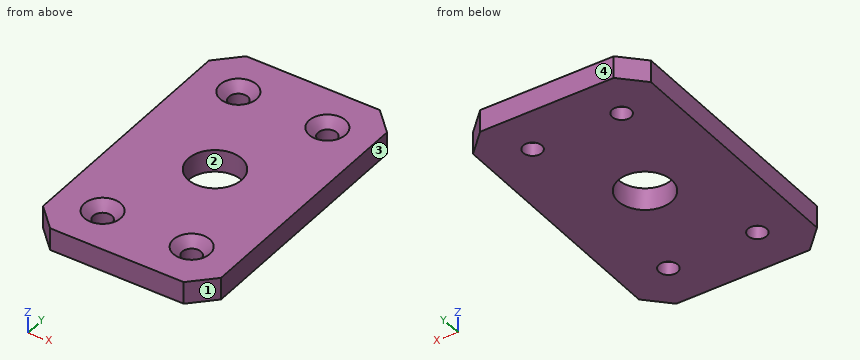
from build123d import *

# Parameters (mm, degrees)
SKETCH_1_W               = 40
SKETCH_1_H               = 65
SKETCH_1_R               = 6
EXTRUDE_1_DEPTH          = 2.5
CUT_EXTRUDE_1_DEPTH      = 39.487010796
CUT_EXTRUDE_1_DEPTH_BACK = 39.487010796
SKETCH_2_R               = 2.1
CHAMFER_1_SIZE           = 2
CHAMFER_2_SIZE           = 5


with BuildPart() as part:
    # 草图1 → 凸台-拉伸1 (new, symmetric)
    with BuildSketch(Plane.XY):
        Rectangle(SKETCH_1_W, SKETCH_1_H)
        Circle(SKETCH_1_R, mode=Mode.SUBTRACT)
    extrude(amount=EXTRUDE_1_DEPTH, both=True)

    # 草图2 → 切除-拉伸1 (cut, two sides: drawn at the far end of the back side and taken through both)
    with BuildSketch(Plane(origin=(0, 0, -2.5), x_dir=(-1, 0, 0), z_dir=(0, 0, -1)).offset(-CUT_EXTRUDE_1_DEPTH_BACK)):
        with Locations((-10, 22.5)):
            Circle(SKETCH_2_R)
        with Locations((10, 22.5)):
            Circle(SKETCH_2_R)
        with Locations((10, -22.5)):
            Circle(SKETCH_2_R)
        with Locations((-10, -22.5)):
            Circle(SKETCH_2_R)
    extrude(amount=CUT_EXTRUDE_1_DEPTH + CUT_EXTRUDE_1_DEPTH_BACK, mode=Mode.SUBTRACT)

    # 倒角1
    chamfer_1_edges = [part.edges().sort_by_distance(p)[0] for p in [
        (12.1, -22.5, 2.5),
        (-7.9, -22.5, 2.5),
        (-7.9, 22.5, 2.5),
        (12.1, 22.5, 2.5),
    ]]
    chamfer(chamfer_1_edges, length=CHAMFER_1_SIZE)

    # 倒角2
    chamfer_2_edges = [part.edges().sort_by_distance(p)[0] for p in [
        (-20, 32.5, 0),
        (20, 32.5, 0),
        (20, -32.5, 0),
        (-20, -32.5, 0),
    ]]
    chamfer(chamfer_2_edges, length=CHAMFER_2_SIZE)


solid = part.part
Check sheet for the modelled part. Datum: model origin and axes. Units: mm. Face numbers are marked on the shaded views. Give positions to 0.01 mm unless a question says otherwise; leave off trailing zeros. Loops run counter-clockwise (first coordinate to the right, second up) from the corner with the lowest first, then second, coordinate; pieces in that order, holes last. Notation, with made-up numbers: M 83,3.25 L 134,3.25 A30 cw 134,35.25 Z; hole C -27,48 d3. An arc over 180 degrees is marked long. Use a Markdown table: item, result. Add a question column.
Q1. Sectioned sample at D-D, the plane z = -1.4. Record the cut outline in (x, y), then the cut area to 3 significant figures.
Q2. Mould release check, pull along Y, two halves, no side actions. Record for the marked faces 1, 2, 3 and 4: pulls with the +Y half, pulls with the -Y half, needs draft (parallel to the pull), parting line crosses it, or undercut.
Q3. Go/stop test with flat-tipped pins: pin 1 (2.5 mm diameter, centred on x = -10, y = -22.5, fed in from -Z); pin 2 (5.5 mm diameter, centred on x = 10, y = 22.5, fed in from -Z). Record where each tip stops, or that it passes through.
Q4. Sectioned sample at B-B, the plane x = -10. Record the cut outline in (y, z).
Q5. Sectioned sample at C-C, the plane y = 0. Record the cut outline in (x, z).
Q6. Scan lines: line 1 along Y through (x, z) = (10, -1.4); line 2 along X through (y, z) = (22.5, -1.75); line 3 along X through (y, z) = (20.5, 1.05). Record each from-to range of solid material in increasing order. Write a range as [from, to].
Q7. Sectioned sample at A-A, the plane x = 0. Record the cut outline in (y, z), then the cut area to 3 significant figures.
Verdict:
| question | item | result |
|---|---|---|
| 1 | outline | M -20,-27.5 L -15,-32.5 L 15,-32.5 L 20,-27.5 L 20,27.5 L 15,32.5 L -15,32.5 L -20,27.5 Z; hole C -10,-22.5 d4.2; hole C -10,22.5 d4.2; hole C 0,0 d12; hole C 10,-22.5 d4.2; hole C 10,22.5 d4.2 |
| 1 | area | 2,380 mm^2 |
| 2 | face 1 | pulls with the -Y half |
| 2 | face 2 | undercut |
| 2 | face 3 | needs draft |
| 2 | face 4 | pulls with the +Y half |
| 3 | pin 1 | through |
| 3 | pin 2 | z = -2.5 |
| 4 | outline | M -32.5,-2.5 L -24.6,-2.5 L -24.6,0.5 L -26.6,2.5 L -32.5,2.5 Z; M -20.4,-2.5 L 20.4,-2.5 L 20.4,0.5 L 18.4,2.5 L -18.4,2.5 L -20.4,0.5 Z; M 24.6,-2.5 L 32.5,-2.5 L 32.5,2.5 L 26.6,2.5 L 24.6,0.5 Z |
| 5 | outline | M -20,-2.5 L -6,-2.5 L -6,2.5 L -20,2.5 Z; M 6,-2.5 L 20,-2.5 L 20,2.5 L 6,2.5 Z |
| 6 | line 1 | [-32.5, -24.6], [-20.4, 20.4], [24.6, 32.5] |
| 6 | line 2 | [-20, -12.1], [-7.9, 7.9], [12.1, 20] |
| 6 | line 3 | [-20, -11.74], [-8.26, 8.26], [11.74, 20] |
| 7 | outline | M -32.5,-2.5 L -6,-2.5 L -6,2.5 L -32.5,2.5 Z; M 6,-2.5 L 32.5,-2.5 L 32.5,2.5 L 6,2.5 Z |
| 7 | area | 265 mm^2 |
